```python
from build123d import *

# Parameters (mm, degrees)
BOSS_EXTRUDE1_DEPTH = 12.5
SKETCH2_R           = 1.4
CUT_EXTRUDE1_DEPTH  = 17.408839081


with BuildPart() as part:
    # Sketch1 → Boss-Extrude1 (new body)
    with BuildSketch(Plane.XY):
        Polygon((0, 0), (8, 0), (8, 7), (0, 7), (0, 5), (6, 5), (6, 2), (0, 2), align=None)
    extrude(amount=BOSS_EXTRUDE1_DEPTH)

    # Sketch2 → Cut-Extrude1 (cut, through all)
    with BuildSketch(Plane(origin=(0, 7, 0), x_dir=(1, 0, 0), z_dir=(0, 1, 0))):
        with Locations(Location((5.8, -6.5, 0), (0, 0, 180))):
            Circle(SKETCH2_R)
    extrude(amount=-CUT_EXTRUDE1_DEPTH, mode=Mode.SUBTRACT)


solid = part.part
```
Geometry check sheet. Reference: the model listing, model coordinates, mm. A direction names the side the tool comes from. Coordinates: 2 decimals unless noted, no trailing zeros. Write each loop counter-clockwise with the first axis right and the second up, starting at its lowest first coordinate (ties: lowest second). Pieces come first, ordered by that corner, then holes. Notation, with made-up numbers: M 15.5,89.5 L 63.5,89.5 A21 cw 63.5,123.5 Z; hole C 14,38 d10. An arc over 180 degrees is marked long. One line per item, written item: value. Start each with the question number.
(1) Sectioned sample at C-C, the plane x = 4. Enter the section's corners in (y, z).
(2) Sectioned sample at A-A, the plane z = 6.5. Enter the section's corners in (x, y).
(3) Depth check by flat-ended pin: pin 1 (0.9 mm diameter, centred on y = 3, z = 9, fed in from -X); pin 2 (1 mm diameter, centred on x = 3.5, y = 3, fed in from +Z). Enter the tip coordinate at first touch or a pass-through.
(4) Sectioned sample at B-B, the plane x = 5.8. Enter the section's corners in (y, z).
(5) Scan lines: line 1 along Y through (x, z) = (1.75, 0.5); line 2 along Z through (x, y) = (5.8, 5.25); line 3 along Z through (x, y) = (6.75, 4.5). Record each from-to range of solid material in increasing order. Write a range as [from, to].
(6) Sectioned sample at D-D, the plane z = 9. Enter the section's corners in (x, y), and give its area (3 significant figures).
(7) Tool access check on faces 3 (the face through (4, 0, 6)), 4 (the face through (6, 4, 10)). Record the directions out of +Z, -Z, +X, -X, +Y, -Y that give a thin tool (end or side, any length) a straight path to the whole face; none if there is none.
(8) Release check for a two-part mould opening along Z. For faces 1 (the face through (3, 2, 6)), 2 (the face through (6.91, 3.55, 5.65)) record: released by +Z, released by -Z, zero draft, split by the parting line, or undercut.
Filled sheet:
1. outline: M 0,0 L 2,0 L 2,12.5 L 0,12.5 Z; M 5,0 L 7,0 L 7,12.5 L 5,12.5 Z
2. outline: M 0,0 L 4.4,0 L 4.4,2 L 0,2 Z; M 0,5 L 4.4,5 L 4.4,7 L 0,7 Z; M 7.2,0 L 8,0 L 8,7 L 7.2,7 Z
3. pin 1: x = 6
3. pin 2: through
4. outline: M 0,0 L 2,0 L 2,5.1 L 0,5.1 Z; M 0,7.9 L 2,7.9 L 2,12.5 L 0,12.5 Z; M 5,0 L 7,0 L 7,5.1 L 5,5.1 Z; M 5,7.9 L 7,7.9 L 7,12.5 L 5,12.5 Z
5. line 1: [0, 2], [5, 7]
5. line 2: [0, 5.1], [7.9, 12.5]
5. line 3: [0, 5.47], [7.53, 12.5]
6. outline: M 0,0 L 8,0 L 8,7 L 0,7 L 0,5 L 6,5 L 6,2 L 0,2 Z
6. area: 38.0 mm²
7. face 3: +Z, -Z, +X, -X, -Y
7. face 4: +Z, -Z, -X
8. face 1: zero draft
8. face 2: undercut
